```python
from build123d import *

# Parameters (mm, degrees)
SKETCH1_W           = 81
SKETCH1_H           = 41
BOSS_EXTRUDE1_DEPTH = 70
SKETCH2_R           = 9.5
CUT_EXTRUDE1_DEPTH  = 115.638562447
SKETCH3_W           = 70
SKETCH3_H           = 4
BOSS_EXTRUDE2_DEPTH = 10
SKETCH4_W           = 70
SKETCH4_H           = 4
BOSS_EXTRUDE3_DEPTH = 10
SKETCH5_R           = 1.4
CUT_EXTRUDE2_DEPTH  = 122.909802723
SKETCH6_W           = 10
SKETCH6_H           = 10
CUT_EXTRUDE3_DEPTH  = 2.5
SKETCH7_W           = 10
SKETCH7_H           = 10
CUT_EXTRUDE4_DEPTH  = 2.5
SKETCH8_W           = 10
SKETCH8_H           = 10
CUT_EXTRUDE5_DEPTH  = 2.5
SKETCH9_W           = 10
SKETCH9_H           = 10
SKETCH9_H_2         = 5
CUT_EXTRUDE6_DEPTH  = 2.5
SKETCH10_R          = 1.4
CUT_EXTRUDE7_DEPTH  = 122.909802723


with BuildPart() as part:
    # Sketch1 → Boss-Extrude1 (new body)
    with BuildSketch(Plane.XY):
        with Locations((40.5, 20.5)):
            Rectangle(SKETCH1_W, SKETCH1_H)
    extrude(amount=BOSS_EXTRUDE1_DEPTH)

    # Sketch2 → Cut-Extrude1 (cut, through all)
    with BuildSketch(Plane.XY.offset(70)):
        with Locations((10.5, 30.5)):
            Circle(SKETCH2_R)
        with Locations((30.5, 30.5)):
            Circle(SKETCH2_R)
        with Locations((50.5, 30.5)):
            Circle(SKETCH2_R)
        with Locations((70.5, 30.5)):
            Circle(SKETCH2_R)
        with Locations((30.5, 10.5)):
            Circle(SKETCH2_R)
        with Locations((50.5, 10.5)):
            Circle(SKETCH2_R)
        with Locations((70.5, 10.5)):
            Circle(SKETCH2_R)
        with Locations((10.5, 10.5)):
            Circle(SKETCH2_R)
    extrude(amount=-CUT_EXTRUDE1_DEPTH, mode=Mode.SUBTRACT)

    # Sketch3 → Boss-Extrude2 (add)
    with BuildSketch(Plane.ZY):
        with Locations((35, 39)):
            Rectangle(SKETCH3_W, SKETCH3_H)
    extrude(amount=BOSS_EXTRUDE2_DEPTH)

    # Sketch4 → Boss-Extrude3 (add)
    with BuildSketch(Plane(origin=(81, 0, 0), x_dir=(0, 0, -1), z_dir=(1, 0, 0))):
        with Locations((-35, 39)):
            Rectangle(SKETCH4_W, SKETCH4_H)
    extrude(amount=BOSS_EXTRUDE3_DEPTH)

    # Sketch5 → Cut-Extrude2 (cut, through all)
    with BuildSketch(Plane(origin=(0, 41, 0), x_dir=(1, 0, 0), z_dir=(0, 1, 0))):
        with Locations(Location((-6, -4, 0), (0, 0, 270))):
            Circle(SKETCH5_R)
        with Locations(Location((-6, -66, 0), (0, 0, 270))):
            Circle(SKETCH5_R)
        with Locations(Location((87, -66, 0), (0, 0, 270))):
            Circle(SKETCH5_R)
        with Locations(Location((87, -4, 0), (0, 0, 270))):
            Circle(SKETCH5_R)
    extrude(amount=-CUT_EXTRUDE2_DEPTH, mode=Mode.SUBTRACT)

    # Sketch6 → Cut-Extrude3 (cut)
    with BuildSketch(Plane.XY.offset(70)):
        with Locations((20.424528373, 30.5)):
            Rectangle(SKETCH6_W, SKETCH6_H)
        with Locations((59.858568815, 30.5)):
            Rectangle(SKETCH6_W, SKETCH6_H)
        with Locations((20.424528373, 10.5)):
            Rectangle(SKETCH6_W, SKETCH6_H)
        with Locations((59.858568815, 10.5)):
            Rectangle(SKETCH6_W, SKETCH6_H)
    extrude(amount=-CUT_EXTRUDE3_DEPTH, mode=Mode.SUBTRACT)

    # Sketch7 → Cut-Extrude4 (cut)
    with BuildSketch(Plane(origin=(0, 0, 0), x_dir=(-1, 0, 0), z_dir=(0, 0, -1))):
        with Locations((-61, 30.5)):
            Rectangle(SKETCH7_W, SKETCH7_H)
        with Locations((-20, 30.5)):
            Rectangle(SKETCH7_W, SKETCH7_H)
        with Locations((-20, 10.5)):
            Rectangle(SKETCH7_W, SKETCH7_H)
        with Locations((-61, 10.5)):
            Rectangle(SKETCH7_W, SKETCH7_H)
    extrude(amount=-CUT_EXTRUDE4_DEPTH, mode=Mode.SUBTRACT)

    # Sketch8 → Cut-Extrude5 (cut)
    with BuildSketch(Plane(origin=(0, 0, 0), x_dir=(-1, 0, 0), z_dir=(0, 0, -1))):
        with Locations((-40, 30.5)):
            Rectangle(SKETCH8_W, SKETCH8_H)
        with Locations((-40, 10.5)):
            Rectangle(SKETCH8_W, SKETCH8_H)
    extrude(amount=-CUT_EXTRUDE5_DEPTH, mode=Mode.SUBTRACT)

    # Sketch9 → Cut-Extrude6 (cut)
    with BuildSketch(Plane.XY.offset(70)):
        with Locations((10.5, 20.5)):
            Rectangle(SKETCH9_W, SKETCH9_H)
        with Locations((79, 30.5)):
            Rectangle(SKETCH9_W, SKETCH9_H_2)
        with Locations((79, 10.5)):
            Rectangle(SKETCH9_W, SKETCH9_H_2)
    extrude(amount=-CUT_EXTRUDE6_DEPTH, mode=Mode.SUBTRACT)

    # Sketch10 → Cut-Extrude7 (cut, through all)
    with BuildSketch(Plane.XY.offset(70)):
        with Locations((20.5, 20.5)):
            Circle(SKETCH10_R)
        with Locations((60.5, 20.5)):
            Circle(SKETCH10_R)
    extrude(amount=-CUT_EXTRUDE7_DEPTH, mode=Mode.SUBTRACT)


solid = part.part
```
Source: CAD feature listing. Evaluate the final solid. Frame: model axes, mm. A direction names the side the tool comes from. Coordinates: 2 decimals unless noted, no trailing zeros. Order: outer loops, then holes, each group sorted by start corner. A loop starts at its lowest first (then second) coordinate and runs counter-clockwise, first axis right, second up. Notation, with made-up numbers: M 34,-9 L 78,-9 A27 ccw 78,16 Z; hole C 31,3 d2. An arc over 180 degrees is marked long. Write each question's results on one line, items separated by ' | '. Start each with the question number.
1) Section query A-A (x = 30.5). Return the cut outline in (y, z).
2) Section query B-B (y = 10.5). Return the cut outline in (x, z), plus the area to 3 significant figures.
3) Access query for faces 1 (the face through (60, 35.5, 69)), 2 (the face through (15.61, 38.51, 35.49)), 3 (the face through (61, 35.5, 1)). Directions: +Z, -Z, +X, -X, +Y, -Y. A direction counts if a zero-diameter tool reaches every point of the face in a straight line with its end or side. Return the directions, or none.
4) Contact query for flat-ended pins moving along their axis: pin 1 Ø5 at (y, z) = (31.5, 38.5) entering from +X; pin 2 Ø10 at (y, z) = (25, 38) entering from -X; pin 3 Ø1.9 at (x, y) = (60.5, 32.5) entering from +Z; pin 4 Ø4 at (x, y) = (65, 32) entering from +Z. Output: stop coordinate, or through.
5) Line query: line 1 (X direction, y = 30.5, z = 26); line 2 (Y direction, x = 50, z = 23); line 3 (Z direction, x = 87, y = 38.65). Output: solid intervals per line, ascending. Write a range as from..to.
6) Section query C-C (z = 35). Give the number of separate pieces and of enclosed holes in the cut face, plus the area to 3 significant figures.
7) Draft query along X for faces 4 (the face through (86, 37, 35)), 5 (the face through (10.4, 20.5, 67.5)). Return one class per face: released by +X, released by -X, zero draft, split by the parting line, or undercut.
Answers:
1) outline: M 0,0 L 1,0 L 1,70 L 0,70 Z; M 20,0 L 21,0 L 21,70 L 20,70 Z; M 40,0 L 41,0 L 41,70 L 40,70 Z
2) outline: M 0,0 L 1,0 L 1,70 L 0,70 Z; M 20,2.5 L 21,2.5 L 21,67.5 L 20,67.5 Z; M 40,2.5 L 41,2.5 L 41,70 L 40,70 Z; M 60,2.5 L 61,2.5 L 61,67.5 L 60,67.5 Z; M 80,0 L 81,0 L 81,67.5 L 80,67.5 Z | area: 335 mm^2
3) face 1: +Z | face 2: +Z, -Z | face 3: -Z
4) pin 1: stops at x = 81 | pin 2: stops at x = 0 | pin 3: stops at z = 67.5 | pin 4: passes through
5) line 1: x = 0..1, 20..21, 40..41, 60..61, 80..81 | line 2: y = 0..1.01, 19.99..21.01, 39.99..41 | line 3: z = 0..2.6, 5.4..64.6, 67.4..70
6) separate pieces: 1 | enclosed holes: 10 | area: 1,120 mm^2
7) face 4: zero draft | face 5: undercut
